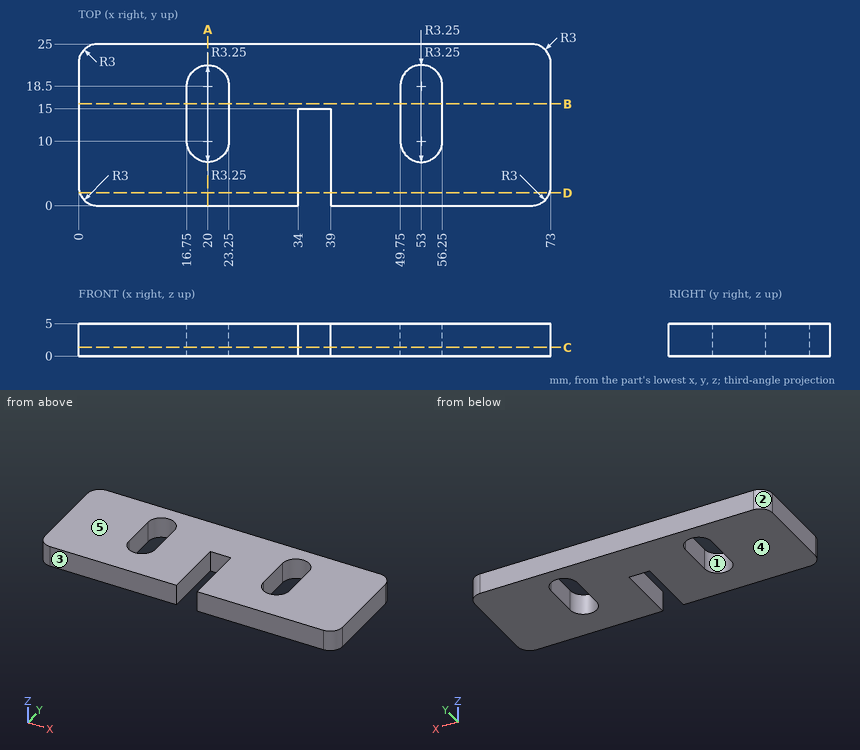
Study the drawing (mm; zero at the part's minimum x, y, z) and answer. A direction names the side the tool comes from. Round coordinates to 2 decimals unless told otherwise and drop trailing zeros. Write each loop counter-clockwise with the first axis right and the second up, starting at its lowest first coordinate (ties: lowest second). Pieces come first, ordered by that corner, then holes.
1) A cutting plane is placed at A-A (x = 20). Give the vertices of the cut face in (y, z), plus the area to 3 significant figures.
2) A tool of negligible diameter and unlimited length cuts with its end or side. For the marked faces 1 and 2, from which of +Z, -Z, +X, -X, +Y, -Y can it reach the whole face along a straight path? Write none if from no direction.
3) Straight lines are drawn through the part: line 1 (X direction, y = 12.75, z = 2.35); line 2 (X direction, y = 17.25, z = 1); line 3 (X direction, y = 21, z = 4.55). For each, find the intervals that lie inside material, in ascending order.
4) A cutting plane is placed at C-C (z = 1.35). Give the vertices of the cut face in (x, y), plus the area to 3 significant figures.
5) A cutting plane is placed at D-D (y = 2). Give the vertices of the cut face in (x, z), plus the area to 3 significant figures.
6) The mould has two halves that part along Z. Classify the marked faces 3, 4 and 5: pulls with the +Z half, pulls with the -Z half, needs draft (parallel to the pull), parting line crosses it, or undercut.
7) Given pin 1 Ø1.5 at (y, z) = (13, 2.5) entering from -X; pin 2 Ø1.5 at (x, z) = (36, 3) entering from -Y, each flat-ended and moving along its own axis, determine where each tip first touches the part or whether it passes through.
8) A cutting plane is placed at B-B (y = 15.75). Give the vertices of the cut face in (x, z).
Completed:
1. outline: (0, 0) - (6.75, 0) - (6.75, 5) - (0, 5) - close; (21.75, 0) - (25, 0) - (25, 5) - (21.75, 5) - close
1. area: 50.0 mm2
2. face 1: +Z, -Z
2. face 2: +Z, -Z, -X, +Y
3. line 1: x = 0 to 16.75, 23.25 to 34, 39 to 49.75, 56.25 to 73
3. line 2: x = 0 to 16.75, 23.25 to 49.75, 56.25 to 73
3. line 3: x = 0 to 17.92, 22.08 to 50.92, 55.08 to 73
4. outline: (0, 3) arc R3 ccw to (3, 0) - (34, 0) - (34, 15) - (39, 15) - (39, 0) - (70, 0) arc R3 ccw to (73, 3) - (73, 22) arc R3 ccw to (70, 25) - (3, 25) arc R3 ccw to (0, 22) - close; hole (16.75, 10) arc R3.25 ccw to (23.25, 10) - (23.25, 18.5) arc R3.25 ccw to (16.75, 18.5) - close; hole (49.75, 10) arc R3.25 ccw to (56.25, 10) - (56.25, 18.5) arc R3.25 ccw to (49.75, 18.5) - close
4. area: 1,570 mm2
5. outline: (0.17, 0) - (34, 0) - (34, 5) - (0.17, 5) - close; (39, 0) - (72.83, 0) - (72.83, 5) - (39, 5) - close
5. area: 338 mm2
6. face 3: needs draft
6. face 4: pulls with the -Z half
6. face 5: pulls with the +Z half
7. pin 1: stops at x = 0
7. pin 2: stops at y = 15
8. outline: (0, 0) - (16.75, 0) - (16.75, 5) - (0, 5) - close; (23.25, 0) - (49.75, 0) - (49.75, 5) - (23.25, 5) - close; (56.25, 0) - (73, 0) - (73, 5) - (56.25, 5) - close
